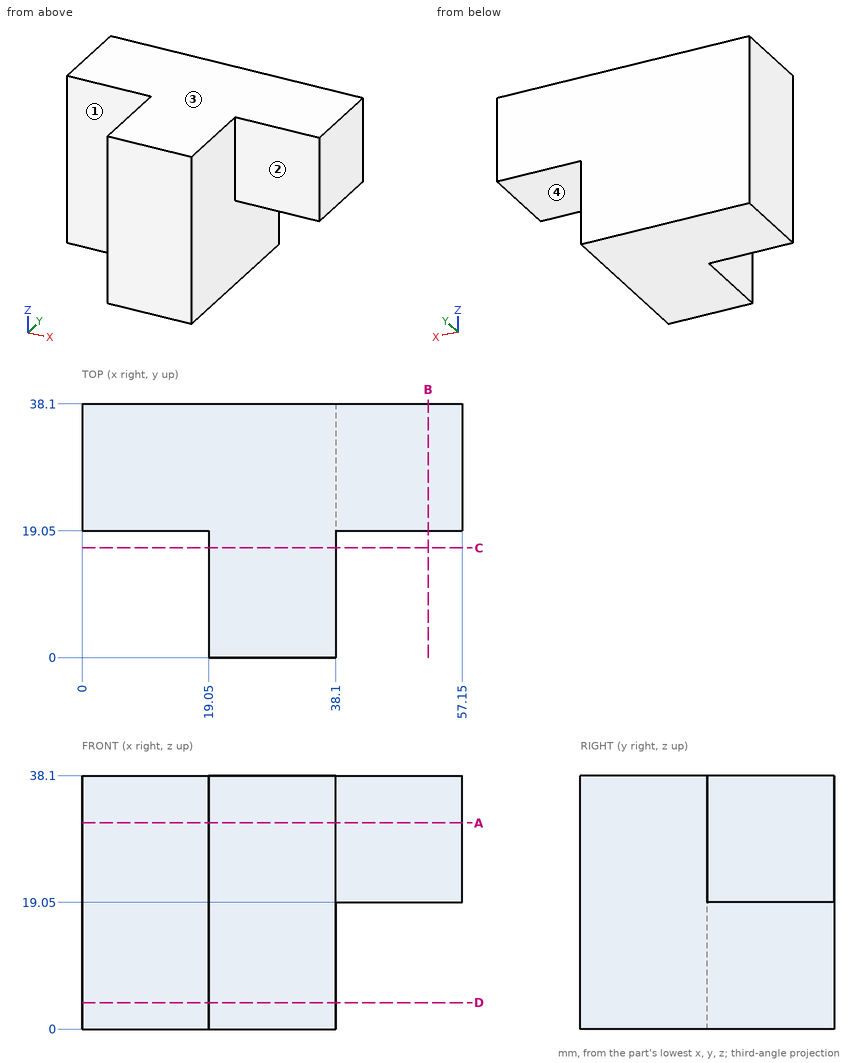
Verification items for this drawing (mm, ordinates from the low corner). A direction names the side the tool comes from. Give positions to 0.01 mm unless a question says otherwise; leave off trailing zeros. Order: outer loops, then holes, each group sorted by start corner. A loop starts at its lowest first (then second) coordinate and runs counter-clockwise, first axis right, second up. Notation, with made-up numbers: M 80,-23 L 96,-23 A15 ccw 96,-15 Z; hole C 21,32.25 d3. An arc over 180 degrees is marked long. Use a Markdown table: item, result.
Item 1: Section check A-A (z = 31). Record the cut outline in (x, y), and give its area (3 significant figures).
Answers follow:
| item | result |
|---|---|
| outline | M 0,19.05 L 19.05,19.05 L 19.05,0 L 38.1,0 L 38.1,19.05 L 57.15,19.05 L 57.15,38.1 L 0,38.1 Z |
| area | 1,450 mm2 |
Item 2: Tool access check on the marked faces 1, 2, 3 and 4. Record the directions out of +Z, -Z, +X, -X, +Y, -Y that give a thin tool (end or side, any length) a straight path to the whole face; none if there is none.
Answers follow:
| item | result |
|---|---|
| face 1 | +Z, -Z, -X, -Y |
| face 2 | +Z, -Z, +X, -Y |
| face 3 | +Z, +X, -X, +Y, -Y |
| face 4 | -Z, +X, +Y, -Y |
Item 3: Material ranges on line 1 along Z through (x, y) = (55, 25.5); line 2 along X through (y, z) = (22.5, 4), recorded low to high.
Answers follow:
| item | result |
|---|---|
| line 1 | z = 19.05 to 38.1 |
| line 2 | x = 0 to 38.1 |
Item 4: Section check C-C (y = 16.5). Record the cut outline in (x, z).
Answers follow:
| item | result |
|---|---|
| outline | M 19.05,0 L 38.1,0 L 38.1,38.1 L 19.05,38.1 Z |
Item 5: Depth check by flat-ended pin: P1, Ø8, axis at y = 15, z = 18.5, coming from the -X side; P2, Ø21, axis at x = 49, z = 31.5, coming from the -Y side; P3, Ø6, axis at x = 50, y = 28, coming from the -Z side. Enter the tip coordinate at first touch or a pass-through.
Answers follow:
| item | result |
|---|---|
| P1 | stops at x = 19.05 |
| P2 | stops at y = 19.05 |
| P3 | stops at z = 19.05 |
Item 6: Section check B-B (x = 52). Record the cut outline in (y, z).
Answers follow:
| item | result |
|---|---|
| outline | M 19.05,19.05 L 38.1,19.05 L 38.1,38.1 L 19.05,38.1 Z |
Item 7: Section check D-D (z = 4). Record the cut outline in (x, y).
Answers follow:
| item | result |
|---|---|
| outline | M 0,19.05 L 19.05,19.05 L 19.05,0 L 38.1,0 L 38.1,38.1 L 0,38.1 Z |
